from build123d import *

# Parameters (mm, degrees)
EXTRUDE_1_DEPTH     = 2.4
SKETCH_2_R          = 2.25
EXTRUDE_2_DEPTH     = 1.4
SKETCH_3_R          = 1.5
CUT_EXTRUDE_1_DEPTH = 4.4


with BuildPart() as part:
    # 草图1 → 凸台-拉伸1 (new body)
    with BuildSketch(Plane.XY):
        Polygon((3.129238459, 0), (1.56461923, 2.71), (-1.56461923, 2.71), (-3.129238459, 0), (-1.56461923, -2.71), (1.56461923, -2.71), align=None)
    extrude(amount=EXTRUDE_1_DEPTH)

    # 草图2 → 凸台-拉伸2 (add)
    with BuildSketch(Plane.XY.offset(2.4)):
        Circle(SKETCH_2_R)
    extrude(amount=EXTRUDE_2_DEPTH)

    # 草图3 → 切除-拉伸1 (cut)
    with BuildSketch(Plane.XY.offset(3.8)):
        Circle(SKETCH_3_R)
    extrude(amount=-CUT_EXTRUDE_1_DEPTH, mode=Mode.SUBTRACT)


solid = part.part
The model under review builds one solid part; all positions refer to its coordinate system, in mm. Round coordinates to 2 decimals unless told otherwise and drop trailing zeros. Write each loop counter-clockwise with the first axis right and the second up, starting at its lowest first coordinate (ties: lowest second). Pieces come first, ordered by that corner, then holes. Notation, with made-up numbers: M 76,-39 L 120,-39 A14 cw 120,-12 Z; hole C 27.5,72 d7. An arc over 180 degrees is marked long. Use a Markdown table: item, result. Add a question column.
Q1. We need section D-D, the plane x = 2.75. State the section outline as (y, z) points, plus the area to 3 significant figures.
Q2. Insertion check: pin 1 (1 mm diameter, centred on y = 0.5, z = 3.5, fed in from -X). The pin has a flat end and moves straight along its axis. Give the tip position at first contact, or say it passes through.
Q3. To check wall thickness, follow line 1 (Y direction, x = 0, z = 0.75); line 2 (Z direction, x = -2, y = -1.8); line 3 (Y direction, x = 0, z = 3.6). State the ranges of each line that lie inside material, in increasing order.
Q4. We need section A-A, the plane x = 0. State the section outline as (y, z) points.
Q5. The part is to be moulded in two halves that separate along X. For faces 1 (the face through (-2.34, 1.37, 1.18)), 2 (the face through (-0.29, 2.23, 3.09)), 3 (the face through (1.3, 1.2, 0)), 4 (the face through (-1.5, 0.07, 1.93)), say which applies: pulls with the +X half, pulls with the -X half, needs draft (parallel to the pull), parting line crosses it, or undercut.
Q6. We need section B-B, the plane z = 0.7. State the section outline as (x, y) points.
Q7. We need section C-C, the plane y = -0.2. State the section outline as (x, z) points.
Findings below:
| question | item | result |
|---|---|---|
| 1 | outline | M -0.66,0 L 0.66,0 L 0.66,2.4 L -0.66,2.4 Z |
| 1 | area | 3.15 mm² |
| 2 | pin 1 | stops at x = -2.25 |
| 3 | line 1 | y = -2.71 to -1.5, 1.5 to 2.71 |
| 3 | line 2 | z = 0 to 2.4 |
| 3 | line 3 | y = -2.25 to -1.5, 1.5 to 2.25 |
| 4 | outline | M -2.71,0 L -1.5,0 L -1.5,3.8 L -2.25,3.8 L -2.25,2.4 L -2.71,2.4 Z; M 1.5,0 L 2.71,0 L 2.71,2.4 L 2.25,2.4 L 2.25,3.8 L 1.5,3.8 Z |
| 5 | face 1 | pulls with the -X half |
| 5 | face 2 | parting line crosses it |
| 5 | face 3 | needs draft |
| 5 | face 4 | undercut |
| 6 | outline | M -3.13,0 L -1.56,-2.71 L 1.56,-2.71 L 3.13,0 L 1.56,2.71 L -1.56,2.71 Z; hole C 0,0 d3 |
| 7 | outline | M -3.01,0 L -1.49,0 L -1.49,3.8 L -2.24,3.8 L -2.24,2.4 L -3.01,2.4 Z; M 1.49,0 L 3.01,0 L 3.01,2.4 L 2.24,2.4 L 2.24,3.8 L 1.49,3.8 Z |
